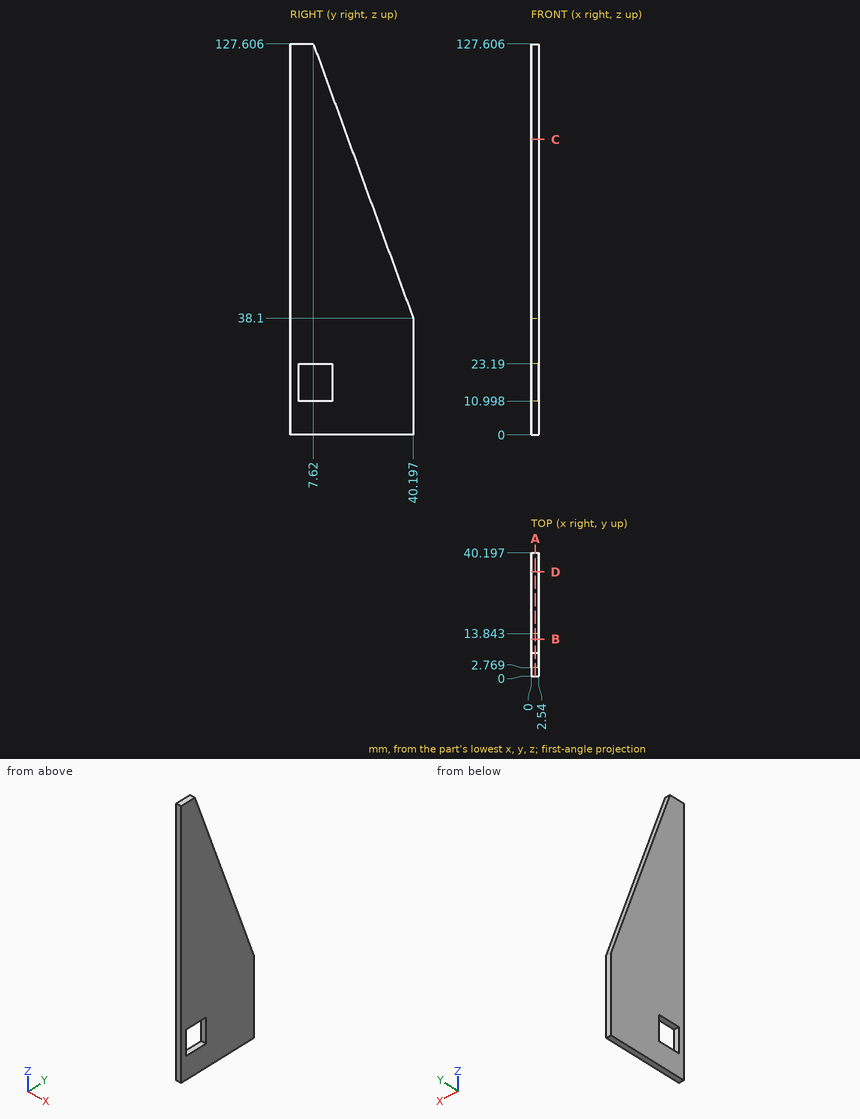
Input: dimensioned drawing with shaded views. Units: mm. Origin: part minimum x, y, z. Coordinates: 2 decimals unless noted, no trailing zeros. Loops run counter-clockwise (first coordinate to the right, second up) from the corner with the lowest first, then second, coordinate; pieces in that order, holes last. Notation, with made-up numbers: M 0,53.25 L 27,53.25 A19 cw 27,68.25 Z; hole C 86.25,14 d9. An arc over 180 degrees is marked long. Use a Markdown table: item, result. Add a question column.
1) Line query: L1, parallel to Z at x = 1.55, y = 7 (1 decimal); L2, parallel to Y at x = 1.9, z = 11.5; L3, parallel to Y at x = 1.8, z = 93 (1 decimal). Output: solid intervals per line, ascending. Write a range as from..to.
2) Section A-A, the plane x = 1.4. Return the cut outline in (y, z) (1 decimal).
3) Section C-C, the plane z = 96.5. Return the cut outline in (x, y), plus the area to 3 significant figures.
4) Section D-D, the plane y = 34. Return the cut outline in (x, z), plus the area to 3 significant figures.
5) Section B-B, the plane y = 12. Return the cut outline in (x, z).
Answer below:
| question | item | result |
|---|---|---|
| 1 | L1 | 0..11, 23.2..127.6 |
| 1 | L2 | 0..2.77, 13.84..40.2 |
| 1 | L3 | 0..20.2 |
| 2 | outline | M 0,0 L 40.2,0 L 40.2,38.1 L 7.6,127.6 L 0,127.6 Z; hole M 2.8,11 L 13.8,11 L 13.8,23.2 L 2.8,23.2 Z |
| 3 | outline | M 0,0 L 2.54,0 L 2.54,18.94 L 0,18.94 Z |
| 3 | area | 48.1 mm2 |
| 4 | outline | M 0,0 L 2.54,0 L 2.54,55.13 L 0,55.13 Z |
| 4 | area | 140 mm2 |
| 5 | outline | M 0,0 L 2.54,0 L 2.54,11 L 0,11 Z; M 0,23.19 L 2.54,23.19 L 2.54,115.57 L 0,115.57 Z |
